Verification items for this drawing (mm, ordinates from the low corner). A direction names the side the tool comes from. Give positions to 0.01 mm unless a question says otherwise; leave off trailing zeros. Loops run counter-clockwise (first coordinate to the right, second up) from the corner with the lowest first, then second, coordinate; pieces in that order, holes last. Notation, with made-up numbers: M -25.75,13 L -8.75,13 A23 ccw -8.75,51 Z; hole C 87.5,-15 d1. An arc over 180 degrees is marked long. Use a Markdown table: item, result.
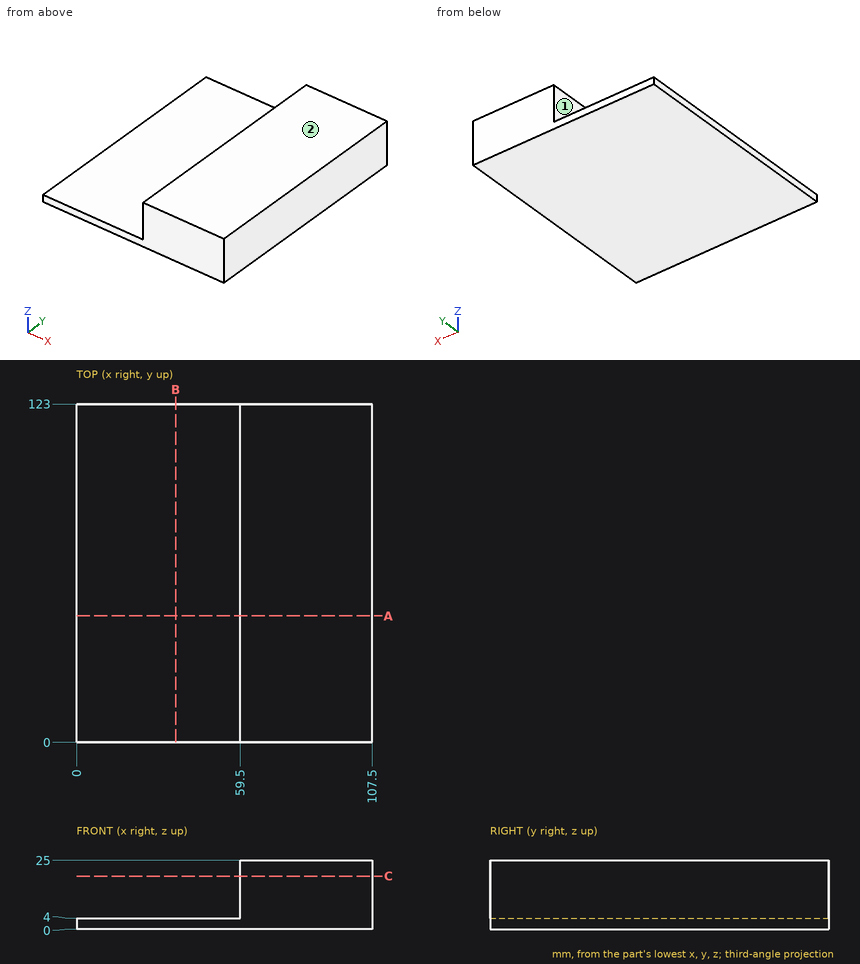
(1) Material ranges on line 1 (X direction, y = 52, z = 8.5); line 2 (Z direction, x = 35.5, y = 54), recorded low to high.
Results below:
| item | result |
|---|---|
| line 1 | 59.5 to 107.5 |
| line 2 | 0 to 4 |
(2) Set-up check for the marked faces 1 and 2: record each of +Z, -Z, +X, -X, +Y, -Y from which the full face is reachable in a straight line by a thin tool's end or side.
Results below:
| item | result |
|---|---|
| face 1 | +Z, -X, +Y, -Y |
| face 2 | +Z, +X, -X, +Y, -Y |
(3) Cross-section at B-B on x = 36. Record the cut outline in (y, z).
Results below:
| item | result |
|---|---|
| outline | M 0,0 L 123,0 L 123,4 L 0,4 Z |
(4) Cross-section at C-C on z = 19.25. Record the cut outline in (x, y).
Results below:
| item | result |
|---|---|
| outline | M 59.5,0 L 107.5,0 L 107.5,123 L 59.5,123 Z |
(5) Cross-section at A-A on y = 46. Record the cut outline in (x, z).
Results below:
| item | result |
|---|---|
| outline | M 0,0 L 107.5,0 L 107.5,25 L 59.5,25 L 59.5,4 L 0,4 Z |
